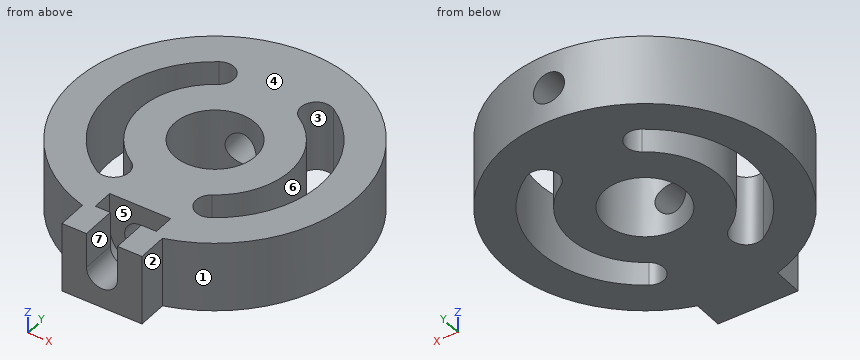
```python
from build123d import *

# Parameters (mm, degrees)
SKETCH_R        = 4.05
EXTRUDE_DEPTH   = 7
SKETCH001_R     = 1.55
POCKET_DEPTH    = 30.723859
POCKET001_DEPTH = 3.5
POCKET002_DEPTH = 2.1


with BuildPart() as part:
    # Sketch → Extrude (new body)
    with BuildSketch(Plane.XY):
        with BuildLine():
            ThreePointArc((4, -13.572859), (0, 14.15), (-4, -13.572859))
            Line((-4, -13.572859), (-4, -16.572859))
            Line((-4, -16.572859), (4, -16.572859))
            Line((4, -16.572859), (4, -13.572859))
        make_face()
        Circle(SKETCH_R, mode=Mode.SUBTRACT)
        with BuildLine():
            ThreePointArc((-4.056612, 6.367605), (-7.55, 0), (-4.056612, -6.367605))
            ThreePointArc((-5.722241, -8.982119), (-3.58217, -8.507677), (-4.056612, -6.367605))
            ThreePointArc((-5.722241, 8.982119), (-10.65, 0), (-5.722241, -8.982119))
            ThreePointArc((-4.056612, 6.367605), (-3.58217, 8.507677), (-5.722241, 8.982119))
        make_face(mode=Mode.SUBTRACT)
        with BuildLine():
            ThreePointArc((4.056612, -6.367605), (7.55, 0), (4.056612, 6.367605))
            ThreePointArc((5.722241, 8.982119), (3.58217, 8.507677), (4.056612, 6.367605))
            ThreePointArc((5.722241, -8.982119), (10.65, 0), (5.722241, 8.982119))
            ThreePointArc((4.056612, -6.367605), (3.58217, -8.507677), (5.722241, -8.982119))
        make_face(mode=Mode.SUBTRACT)
    extrude(amount=EXTRUDE_DEPTH)

    # Sketch001 → Pocket (cut, through all)
    with BuildSketch(Plane.XZ.offset(16.572859)):
        with Locations((0, 3.5)):
            Circle(SKETCH001_R)
    extrude(amount=-POCKET_DEPTH, mode=Mode.SUBTRACT)

    # Sketch002 → Pocket001 (cut)
    with BuildSketch(Plane.XY.offset(7)):
        Polygon((-3.049999, -10.972859), (-3.049999, -13.072859), (-1.549999, -13.072859), (-1.549999, -16.572859), (1.550001, -16.572859), (1.550001, -13.072859), (3.050001, -13.072859), (3.050001, -10.972859), align=None)
    extrude(amount=-POCKET001_DEPTH, mode=Mode.SUBTRACT)

    # Sketch003 → Pocket002 (cut)
    with BuildSketch(Plane.XZ.offset(10.972859)):
        with BuildLine():
            ThreePointArc((-3.050001, 3.5), (0, 0.449999), (3.050001, 3.5))
            Line((-3.050001, 3.5), (3.050001, 3.5))
        make_face()
    extrude(amount=POCKET002_DEPTH, mode=Mode.SUBTRACT)


solid = part.part
```
The listing builds one solid part. Answer for the finished solid, in the listing's coordinates (mm). Face numbers are marked on the shaded views. A direction names the side the tool comes from. Coordinates: 2 decimals unless noted, no trailing zeros. Write each loop counter-clockwise with the first axis right and the second up, starting at its lowest first coordinate (ties: lowest second). Pieces come first, ordered by that corner, then holes. Notation, with made-up numbers: M 11,-36 L 38,-36 A19 ccw 38,-6 Z; hole C 14,36 d3. An arc over 180 degrees is marked long. Use a Markdown table: item, result. Add a question column.
1. Given P1, Ø1.5, axis at y = -15, z = 3, coming from the +X side; P2, Ø2.5, axis at y = -12, z = 5, coming from the +X side; P3, Ø3.5, axis at y = -14.5, z = 2, coming from the -X side, each flat-ended and moving along its own axis, determine where each tip first touches the part or whether it passes through.
2. Section B-B (x = 0) is taken. Give the vertices of the cut face in (y, z).
3. Section A-A (y = 0) is taken. Give the vertices of the cut face in (x, z), plus the area to 3 significant figures.
4. Which of the six approach directions +Z, -Z, +X, -X, +Y, -Y give full straight-line access (tool end or side, diameter ignored) to the marked faces 4, 5, 6 and 7?
5. Section D-D (y = 5) is taken. Give the vertices of the cut face in (x, z), plus the area to 3 significant figures.
6. Straight lines are drawn through the part: line 1 along Y through (x, z) = (0, 1.5); line 2 along Z through (x, y) = (0, 10); line 3 along X through (y, z) = (-8, 3.5). For each, find the intervals that lie inside material, in ascending order. Write a range as [from, to].
7. For a pull along X with two mould halves and no side action, classify the marked faces 1, 2 and 3 as +X half, -X half, draft (parallel to the pull), parting line (faces both ways), or undercut.
8. Section C-C (z = 6.5) is taken. Give the vertices of the cut face in (x, y), plus the area to 3 significant figures.
Data:
| question | item | result |
|---|---|---|
| 1 | P1 | stops at x = 4 |
| 1 | P2 | stops at x = 9.2 |
| 1 | P3 | stops at x = -6.14 |
| 2 | outline | M -16.57,0 L -4.05,0 L -4.05,1.95 L -10.97,1.95 L -10.97,0.45 L -13.07,0.45 L -13.07,1.95 L -16.57,1.95 Z; M -10.97,5.05 L -4.05,5.05 L -4.05,7 L -10.97,7 Z; M 4.05,0 L 14.15,0 L 14.15,1.95 L 4.05,1.95 Z; M 4.05,5.05 L 14.15,5.05 L 14.15,7 L 4.05,7 Z |
| 3 | outline | M -14.15,0 L -10.65,0 L -10.65,7 L -14.15,7 Z; M -7.55,0 L -4.05,0 L -4.05,7 L -7.55,7 Z; M 4.05,0 L 7.55,0 L 7.55,7 L 4.05,7 Z; M 10.65,0 L 14.15,0 L 14.15,7 L 10.65,7 Z |
| 3 | area | 98.0 mm2 |
| 4 | face 4 | +Z, +X, -X, +Y, -Y |
| 4 | face 5 | +Z |
| 4 | face 6 | +Z, -Z |
| 4 | face 7 | +Z, -Y |
| 5 | outline | M -13.24,0 L -9.4,0 L -9.4,7 L -13.24,7 Z; M -5.66,0 L 5.66,0 L 5.66,7 L -5.66,7 Z; M 9.4,0 L 13.24,0 L 13.24,7 L 9.4,7 Z; hole C 0,3.5 d3.1 |
| 5 | area | 125 mm2 |
| 6 | line 1 | y = [-16.57, -13.07], [-10.97, -4.05], [4.05, 14.15] |
| 6 | line 2 | z = [0, 1.95], [5.05, 7] |
| 6 | line 3 | x = [-11.67, -7.03], [-3.37, -1.55], [1.55, 3.37], [7.03, 11.67] |
| 7 | face 1 | parting line |
| 7 | face 2 | +X half |
| 7 | face 3 | undercut |
| 8 | outline | M -4,-16.57 L -1.55,-16.57 L -1.55,-13.07 L -3.05,-13.07 L -3.05,-10.97 L 3.05,-10.97 L 3.05,-13.07 L 1.55,-13.07 L 1.55,-16.57 L 4,-16.57 L 4,-13.57 A14.15 ccw long -4,-13.57 Z; hole M -5.72,-8.98 A1.55 ccw -4.06,-6.37 A7.55 cw -4.06,6.37 A1.55 ccw -5.72,8.98 A10.65 ccw Z; hole C 0,0 d8.1; hole M 4.06,-6.37 A1.55 ccw 5.72,-8.98 A10.65 ccw 5.72,8.98 A1.55 ccw 4.06,6.37 A7.55 cw Z |
| 8 | area | 446 mm2 |
